Model file for the job. Use its own axes, mm. Round coordinates to 2 decimals unless told otherwise and drop trailing zeros. Order: outer loops, then holes, each group sorted by start corner. A loop starts at its lowest first (then second) coordinate and runs counter-clockwise, first axis right, second up. Notation, with made-up numbers: (29, 40) -> (49, 40) arc R32 ccw to (49, 75) -> close; hole circle Ø10 at (-38.75, 59). An arc over 180 degrees is marked (long way). Put each result on its own line as item: value. Start each with the question number.
Q1. Cut at A-A, the plane x = 0. List the corners of the cut face in (y, z).
Q2. Probe L1, parallel to Z at x = -15, y = -4.35; L2, parallel to X at y = -2.45, z = -11; L3, parallel to Y at x = 0, z = 12. List the from-to ranges inside material, lowest first.
Q3. Cut at D-D, the plane x = -15. List the corners of the cut face in (y, z), and give its area (3 significant figures).
Q4. Cut at C-C, the plane y = -1.4. List the corners of the cut face in (x, z).
Q5. Flat gauge pins, fed straight in: P1, Ø5, axis at x = -15, z = -10, coming from the -Y side; P2, Ø4, axis at x = 0, z = 5, coming from the +Y side. Where does each tip first touch, or does it go through?
Q6. Cut at B-B, the plane z = -10. List the corners of the cut face in (x, y), and give its area (3 significant figures).
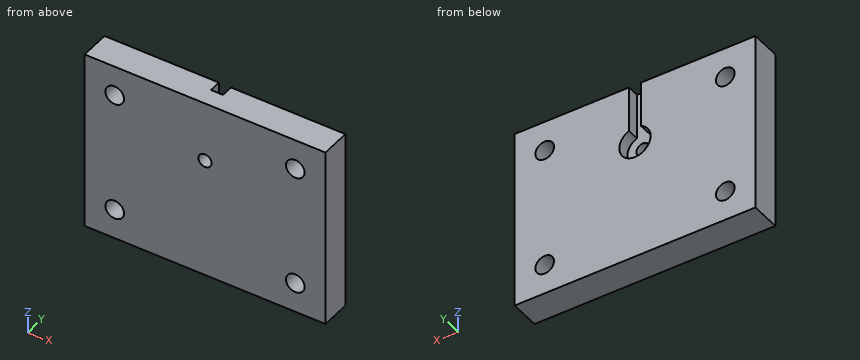
from build123d import *

# Parameters (mm, degrees)
F0_R     = 1.55
F0_R_2   = 1.1
F1_DEPTH = 5
F2_DEPTH = 2


with BuildPart() as f1:
    # F0 (on Front) → F1 (new body)
    with BuildSketch(Plane.XZ):
        with BuildLine():
            Line((-20, -15), (20, -15))
            Line((20, -15), (20, 15))
            Line((20, 15), (1, 15))
            Line((1, 15), (1, 7.4))
            ThreePointArc((1, 7.4), (0, 2.4), (-1, 7.4))
            Line((-1, 7.4), (-1, 15))
            Line((-1, 15), (-20, 15))
            Line((-20, 15), (-20, -15))
        make_face()
        with Locations((-15, -10)):
            Circle(F0_R, mode=Mode.SUBTRACT)
        with Locations((15, -10)):
            Circle(F0_R, mode=Mode.SUBTRACT)
        with Locations((-15, 10)):
            Circle(F0_R, mode=Mode.SUBTRACT)
        with Locations((15, 10)):
            Circle(F0_R, mode=Mode.SUBTRACT)
        with BuildLine():
            Line((1, 7.4), (1, 15))
            Line((1, 15), (-1, 15))
            Line((-1, 15), (-1, 7.4))
            ThreePointArc((-1, 7.4), (0, 2.4), (1, 7.4))
        make_face()
        with Locations((0, 5)):
            Circle(F0_R_2, mode=Mode.SUBTRACT)
    extrude(amount=F1_DEPTH)

    # F0 (on Front) → F2 (cut)
    with BuildSketch(Plane.XZ):
        with BuildLine():
            Line((1, 7.4), (1, 15))
            Line((1, 15), (-1, 15))
            Line((-1, 15), (-1, 7.4))
            ThreePointArc((-1, 7.4), (0, 2.4), (1, 7.4))
        make_face()
        with Locations((0, 5)):
            Circle(F0_R_2, mode=Mode.SUBTRACT)
    extrude(amount=F2_DEPTH, mode=Mode.SUBTRACT)


solid = f1.part
Ans:
1. outline: (-5, -15) -> (0, -15) -> (0, 2.4) -> (-2, 2.4) -> (-2, 3.9) -> (-5, 3.9) -> close; (-5, 6.1) -> (-2, 6.1) -> (-2, 15) -> (-5, 15) -> close
2. L1: z = -15 to -11.55, -8.45 to 8.45, 11.55 to 15
2. L2: x = -20 to -16.18, -13.82 to 13.82, 16.18 to 20
2. L3: y = -5 to -2
3. outline: (-5, -15) -> (0, -15) -> (0, -11.55) -> (-5, -11.55) -> close; (-5, -8.45) -> (0, -8.45) -> (0, 8.45) -> (-5, 8.45) -> close; (-5, 11.55) -> (0, 11.55) -> (0, 15) -> (-5, 15) -> close
3. area: 119 mm^2
4. outline: (-20, -15) -> (20, -15) -> (20, 15) -> (1, 15) -> (1, 7.4) arc R2.6 cw (long way) to (-1, 7.4) -> (-1, 15) -> (-20, 15) -> close; hole circle Ø3.1 at (-15, -10); hole circle Ø3.1 at (-15, 10); hole circle Ø3.1 at (15, -10); hole circle Ø3.1 at (15, 10)
5. P1: stops at y = -5
5. P2: stops at y = -2
6. outline: (-20, -5) -> (-16.55, -5) -> (-16.55, 0) -> (-20, 0) -> close; (-13.45, -5) -> (13.45, -5) -> (13.45, 0) -> (-13.45, 0) -> close; (16.55, -5) -> (20, -5) -> (20, 0) -> (16.55, 0) -> close
6. area: 169 mm^2
